Verification items for the finished model (mm, model axes). A direction names the side the tool comes from. Give positions to 0.01 mm unless a question says otherwise; leave off trailing zeros. Write each loop counter-clockwise with the first axis right and the second up, starting at its lowest first coordinate (ties: lowest second). Pieces come first, ordered by that corner, then holes. Notation, with made-up numbers: M 55,35.25 L 69,35.25 A19 cw 69,58.25 Z; hole C 78.5,41.5 d7. An arc over 180 degrees is marked long. Answer as a JSON object with one key per item and string values.
```python
from build123d import *

# Parameters (mm, degrees)
F0_W           = 50
F0_H           = 210
F1_DEPTH       = 12
F3_D           = 8.8
F3_CSINK_D     = 17.92
F3_CSINK_ANGLE = 90
F5_D           = 15
F7_D           = 5
F7_DEPTH       = 20
F7_TIP         = 1.5021515476


with BuildPart() as f1:
    # F0 (on Top) → F1 (new body)
    with BuildSketch(Plane.XY):
        with Locations((25, 105)):
            Rectangle(F0_W, F0_H)
    extrude(amount=-F1_DEPTH)

    # F3 (through all)
    with Locations(Plane.XY):
        with Locations((12.5, 20), (37.5, 20), (37.5, 190), (12.5, 190)):
            CounterSinkHole(F3_D / 2, F3_CSINK_D / 2, counter_sink_angle=F3_CSINK_ANGLE)

    # F5 (through all)
    with Locations(Plane.XY):
        with Locations((25, 105)):
            Hole(F5_D / 2)

    # F7
    with Locations(Plane(origin=(0, 0, 0), x_dir=(0, -1, 0), z_dir=(-1, 0, 0))):
        with Locations((-105, -6)):
            Hole(F7_D / 2, depth=F7_DEPTH)
            with Locations((0, 0, -(F7_DEPTH + F7_TIP / 2))):  # 118° drill point
                Cone(0, F7_D / 2, F7_TIP, mode=Mode.SUBTRACT)


solid = f1.part
```
1) Release check for a two-part mould opening along Y. For faces 1 (the face through (50, 104, -6)), 2 (the face through (8.303, 21.322, -8.332)), 3 (the face through (25, 0, -6)) record: pulls with the +Y half, pulls with the -Y half, needs draft (parallel to the pull), parting line crosses it, or undercut.
Completed:
{"face 1": "needs draft", "face 2": "undercut", "face 3": "pulls with the -Y half"}
2) Section check A-A on x = 25. Record the boundary of the cut face in (y, z).
Completed:
{"outline": "M 0,-12 L 97.5,-12 L 97.5,0 L 0,0 Z; M 112.5,-12 L 210,-12 L 210,0 L 112.5,0 Z"}
3) Section check C-C on x = 37.5. Record the boundary of the cut face in (y, z).
Completed:
{"outline": "M 0,-12 L 15.6,-12 L 15.6,-4.56 L 11.04,0 L 0,0 Z; M 24.4,-12 L 185.6,-12 L 185.6,-4.56 L 181.04,0 L 28.96,0 L 24.4,-4.56 Z; M 194.4,-12 L 210,-12 L 210,0 L 198.96,0 L 194.4,-4.56 Z"}
4) Section check B-B on y = 20. Record the boundary of the cut face in (x, z), and give its area (3 significant figures).
Completed:
{"outline": "M 0,-12 L 8.1,-12 L 8.1,-4.56 L 3.54,0 L 0,0 Z; M 16.9,-12 L 33.1,-12 L 33.1,-4.56 L 28.54,0 L 21.46,0 L 16.9,-4.56 Z; M 41.9,-12 L 50,-12 L 50,0 L 46.46,0 L 41.9,-4.56 Z", "area": "347 mm2"}
5) Thickness scan on L1, parallel to X at y = 20, z = -8.5; L2, parallel to Y at x = 12.5, z = -9.75; L3, parallel to Y at x = 25, z = -5.5. Record the ranges inside material, lowest first.
Completed:
{"L1": "x = 0 to 8.1, 16.9 to 33.1, 41.9 to 50", "L2": "y = 0 to 15.6, 24.4 to 185.6, 194.4 to 210", "L3": "y = 0 to 97.5, 112.5 to 210"}
6) Access from +Z, -Z, +X, -X, +Y, -Y to the whole of each face (thin tool, end or side, straight path). Record for faces 4 (the face through (9.09, 107.385, -5.249)), 5 (the face through (13.5, 185.49, -4.34)).
Completed:
{"face 4": "-X", "face 5": "+Z"}
7) Go/stop test with flat-tipped pins: pin 1 (14 mm diameter, centred on x = 12.5, y = 190, fed in from +Z); pin 2 (11.5 mm diameter, centred on x = 12.5, y = 20, fed in from +Z); pin 3 (7 mm diameter, centred on x = 37.5, y = 20, fed in from -Z). Record where each tip stops, or that it passes through.
Completed:
{"pin 1": "stops at z = -1.96", "pin 2": "stops at z = -3.21", "pin 3": "passes through"}
